Geometry check sheet. Reference: the model listing, model coordinates, mm. A direction names the side the tool comes from. Round coordinates to 2 decimals unless told otherwise and drop trailing zeros. Write each loop counter-clockwise with the first axis right and the second up, starting at its lowest first coordinate (ties: lowest second). Pieces come first, ordered by that corner, then holes. Notation, with made-up numbers: (55, 35) -> (93, 35) arc R17 ccw to (93, 50) -> close; hole circle Ø9 at (16.25, 85). An arc over 180 degrees is marked (long way). One line per question, with ' | ' between items.
```python
from build123d import *

# Parameters (mm, degrees)
BOSS_EXTRUDE2_DEPTH = 120
SHELL2_T            = -2
SKETCH12_W          = 12
SKETCH12_H          = 10
CUT_EXTRUDE4_DEPTH  = 5
CUT_EXTRUDE8_REACH  = 122
SKETCH22_R          = 1.58
SKETCH22_R_2        = 10
BOSS_EXTRUDE4_DEPTH = 30
CUT_EXTRUDE9_REACH  = 122
SKETCH27_W          = 2
SKETCH27_H          = 2
BOSS_EXTRUDE5_DEPTH = 2


with BuildPart() as part:
    # Sketch1 → Boss-Extrude2 (new body)
    with BuildSketch(Plane(origin=(0, 0, 0), x_dir=(1, 0, 0), z_dir=(0, 1, 0))):
        with BuildLine():
            Line((-77.5, -23.128972286), (62.5, -23.128972286))
            ThreePointArc((62.5, -23.128972286), (84.701532545, 38.031487477), (32.5, 76.871027714))
            Line((32.5, 76.871027714), (-47.5, 76.871027714))
            ThreePointArc((-47.5, 76.871027714), (-99.701532545, 38.031487477), (-77.5, -23.128972286))
        make_face()
    extrude(amount=BOSS_EXTRUDE2_DEPTH)

    # Shell2
    shell2_openings = [part.faces().sort_by_distance(p)[0] for p in [
        (-7.5, 120, -32.451257595),
    ]]
    offset(amount=SHELL2_T, openings=shell2_openings, kind=Kind.INTERSECTION)

    # Sketch12 → Cut-Extrude4 (cut)
    with BuildSketch(Plane(origin=(0, 2, 0), x_dir=(1, 0, 0), z_dir=(0, 1, 0))):
        with Locations((55.893876913, -9.063838959)):
            Rectangle(SKETCH12_W, SKETCH12_H)
    extrude(amount=-CUT_EXTRUDE4_DEPTH, mode=Mode.SUBTRACT)

    # Sketch22 → Cut-Extrude8 (cut, up to next)
    with BuildSketch(Plane(origin=(0, 0, 0), x_dir=(1, 0, 0), z_dir=(0, 1, 0)), mode=Mode.PRIVATE) as cut_extrude8_sk1:
        with Locations((-67.5, -16.628972286)):
            Circle(SKETCH22_R)
    cut_extrude8_tool1 = extrude(cut_extrude8_sk1.sketch, amount=CUT_EXTRUDE8_REACH, mode=Mode.PRIVATE) & part.part
    add(cut_extrude8_tool1.solids().sort_by_distance((-67.5, 0, 16.628972))[0], mode=Mode.SUBTRACT)
    # Sketch22 → Cut-Extrude8 (cut, up to next)
    with BuildSketch(Plane(origin=(0, 0, 0), x_dir=(1, 0, 0), z_dir=(0, 1, 0)), mode=Mode.PRIVATE) as cut_extrude8_sk2:
        with Locations((-67.5, 47.344907447)):
            Circle(SKETCH22_R)
    cut_extrude8_tool2 = extrude(cut_extrude8_sk2.sketch, amount=CUT_EXTRUDE8_REACH, mode=Mode.PRIVATE) & part.part
    add(cut_extrude8_tool2.solids().sort_by_distance((-67.5, 0, -47.344907))[0], mode=Mode.SUBTRACT)
    # Sketch22 → Cut-Extrude8 (cut, up to next)
    with BuildSketch(Plane(origin=(0, 0, 0), x_dir=(1, 0, 0), z_dir=(0, 1, 0)), mode=Mode.PRIVATE) as cut_extrude8_sk3:
        with Locations((-32.5, 26.344907447)):
            Circle(SKETCH22_R_2)
    cut_extrude8_tool3 = extrude(cut_extrude8_sk3.sketch, amount=CUT_EXTRUDE8_REACH, mode=Mode.PRIVATE) & part.part
    add(cut_extrude8_tool3.solids().sort_by_distance((-32.5, 0, -26.344907))[0], mode=Mode.SUBTRACT)

    # Sketch23 → Boss-Extrude4 (add)
    with BuildSketch(Plane(origin=(0, 0, 0), x_dir=(1, 0, 0), z_dir=(0, 1, 0))):
        Polygon((51.893876913, 46.61041607), (51.893876913, 0.61041607), (69.893876913, 0.61041607), (69.893876913, 46.61041607), (71.893876913, 46.61041607), (71.893876913, -1.38958393), (49.893876913, -1.38958393), (49.893876913, 46.61041607), align=None)
    extrude(amount=BOSS_EXTRUDE4_DEPTH)

    # Sketch24 → Cut-Extrude9 (cut, up to next)
    with BuildSketch(Plane(origin=(0, 0, 0), x_dir=(1, 0, 0), z_dir=(0, 1, 0)), mode=Mode.PRIVATE) as cut_extrude9_sk1:
        with BuildLine():
            Line((54.893876913, 56.61041607), (66.893876913, 56.61041607))
            ThreePointArc((66.893876913, 56.61041607), (70.429410819, 55.145949976), (71.893876913, 51.61041607))
            Line((71.893876913, 51.61041607), (71.893876913, 46.61041607))
            Line((71.893876913, 46.61041607), (69.893876913, 46.61041607))
            Line((69.893876913, 46.61041607), (69.893876913, 41.61041607))
            Line((69.893876913, 41.61041607), (51.893876913, 41.61041607))
            Line((51.893876913, 41.61041607), (51.893876913, 46.61041607))
            Line((51.893876913, 46.61041607), (49.893876913, 46.61041607))
            Line((49.893876913, 46.61041607), (49.893876913, 51.61041607))
            ThreePointArc((49.893876913, 51.61041607), (51.358343007, 55.145949976), (54.893876913, 56.61041607))
        make_face()
    cut_extrude9_tool1 = extrude(cut_extrude9_sk1.sketch, amount=CUT_EXTRUDE9_REACH, mode=Mode.PRIVATE) & part.part
    add(cut_extrude9_tool1.solids().sort_by_distance((60.893877, 0, -49.215699))[0], mode=Mode.SUBTRACT)

    # Sketch27 → Boss-Extrude5 (add)
    with BuildSketch(Plane(origin=(0, 120, 0), x_dir=(1, 0, 0), z_dir=(0, 1, 0))):
        with Locations((-46.5, 75.871027714)):
            Rectangle(SKETCH27_W, SKETCH27_H)
        with Locations((31.5, 75.871027714)):
            Rectangle(SKETCH27_W, SKETCH27_H)
        with Locations((60.893876913, -22.128972286)):
            Rectangle(SKETCH27_W, SKETCH27_H)
        with Locations((-75.893876913, -22.128972286)):
            Rectangle(SKETCH27_W, SKETCH27_H)
    extrude(amount=BOSS_EXTRUDE5_DEPTH)


solid = part.part
```
(1) Sectioned sample at A-A on y = 27. Record the cut outline in (x, z).
Resolved:
outline: (-77.5, 23.13) arc R54.5 ccw to (-47.5, -76.87) -> (32.5, -76.87) arc R54.5 ccw to (62.5, 23.13) -> close; (49.89, -46.61) -> (51.89, -46.61) -> (51.89, -0.61) -> (69.89, -0.61) -> (69.89, -46.61) -> (71.89, -46.61) -> (71.89, 1.39) -> (49.89, 1.39) -> close; hole (-76.89, 21.13) arc R52.5 ccw to (-47.5, -74.87) -> (32.5, -74.87) arc R52.5 ccw to (61.89, 21.13) -> close
(2) Sectioned sample at B-B on x = -32.5. Record the cut outline in (y, z), then the cut area to 3 significant figures.
Resolved:
outline: (0, -76.87) -> (120, -76.87) -> (120, -74.87) -> (2, -74.87) -> (2, -36.34) -> (0, -36.34) -> close; (0, -16.34) -> (2, -16.34) -> (2, 21.13) -> (120, 21.13) -> (120, 23.13) -> (0, 23.13) -> close | area: 632 mm2
(3) Go/stop test with flat-tipped pins: pin 1 (24 mm diameter, centred on x = 58, z = -16.5, fed in from +Y); pin 2 (2 mm diameter, centred on y = 121.5, z = -76, fed in from +X); pin 3 (6 mm diameter, centred on y = 38.5, z = -26.5, fed in from -X). Record where each tip stops, or that it passes through.
Resolved:
pin 1: stops at y = 30 | pin 2: stops at x = 32.5 | pin 3: stops at x = -101.99
(4) Sectioned sample at C-C on y = 101. Record the cut outline in (x, z).
Resolved:
outline: (-77.5, 23.13) arc R54.5 ccw to (-47.5, -76.87) -> (32.5, -76.87) arc R54.5 ccw to (62.5, 23.13) -> close; hole (-76.89, 21.13) arc R52.5 ccw to (-47.5, -74.87) -> (32.5, -74.87) arc R52.5 ccw to (61.89, 21.13) -> close
(5) Access from +Z, -Z, +X, -X, +Y, -Y to the whole of each face (thin tool, end or side, straight path). Record for faces 1 (the flat face through (71, 30, -19)), 2 (the cylindrical face through (51.32, 0.99, -55.11)), 3 (the flat face through (-8, 60, -76.871)).
Resolved:
face 1: +Y | face 2: +Y, -Y | face 3: -Z, +X, -X, +Y, -Y
(6) Material ranges on line 1 (Z direction, x = 27, y = 84); line 2 (Z direction, x = -67.5, y = 0.4); line 3 (Z direction, x = -32.5, y = 0.9), recorded low to high.
Resolved:
line 1: z = -76.87 to -74.87, 21.13 to 23.13 | line 2: z = -73.07 to -48.92, -45.76 to 15.05, 18.21 to 23.13 | line 3: z = -76.87 to -36.34, -16.34 to 23.13
(7) Draft check along Z on faces 4 (the flat face through (-97, 120, -42)), 5 (the flat face through (-8, 61, 21.129)), 6 (the cylindrical face through (-99.4, 59.2, -39)). Enter one of: +Z half, -Z half, draft (parallel to the pull), parting line (faces both ways), or undercut.
Resolved:
face 4: draft | face 5: undercut | face 6: parting line
(8) Sectioned sample at D-D on z = -67. Record the cut outline in (x, y), then the cut area to 3 significant figures.
Resolved:
outline: (-78.78, 0) -> (63.78, 0) -> (63.78, 120) -> (60.15, 120) -> (60.15, 2) -> (-75.15, 2) -> (-75.15, 120) -> (-78.78, 120) -> close | area: 1,140 mm2
